Here's how the part is built. I have some questions about the finished solid (model axes, mm). A direction names the side the tool comes from. Give positions to 0.01 mm unless a question says otherwise; leave off trailing zeros. Write each loop counter-clockwise with the first axis right and the second up, starting at its lowest first coordinate (ties: lowest second). Pieces come first, ordered by that corner, then holes. Notation, with made-up numbers: (-21.5, -1) - (35.5, -1) arc R36 cw to (35.5, 37) - close; hole circle Ø4 at (74.5, 52). An arc over 180 degrees is marked (long way). Use one line per item in the form item = value. Start each with the question number.
from build123d import *

# Parameters (mm, degrees)
F1_DEPTH = 177.8
F2_R     = 12.7
F3_R     = 3.17499


# Not quite as in the source:
# - a fillet or chamfer is up to 0.001 mm smaller than in the source, because OpenCascade refuses the exact size


with BuildPart() as f1:
    # F0 (on Right) → F1 (new body, symmetric)
    with BuildSketch(Plane.YZ):
        Polygon((70.9975426912, -81.0872844047), (70.9975426912, 71.3127155953), (-81.4024573088, 71.3127155953), (-81.4024573088, -38.3387617767), (-62.3524573088, -49.3372844047), (-62.3524573088, -74.7372844047), (-81.4024573088, -74.7372844047), (-81.4024573088, -81.0872844047), align=None)
    extrude(amount=F1_DEPTH, both=True)

    # F2
    f2_edges = [f1.edges().sort_by_distance(p)[0] for p in [
        (0, -81.402457, -38.338762),
        (0, -81.402457, 71.312716),
        (0, 70.997543, 71.312716),
        (0, 70.997543, -81.087284),
    ]]
    fillet(f2_edges, radius=F2_R)

    # F3 (radius 3.175 in the source; OpenCascade refuses exactly that, so slightly less here)
    f3_edges = [f1.edges().sort_by_distance(p)[0] for p in [
        (0, -81.402457, -74.737284),
        (0, -81.402457, -81.087284),
    ]]
    fillet(f3_edges, radius=F3_R)


solid = f1.part
1. Please list where these lines run through material, in increasing order: line 1 (Y direction, x = -132.5, z = -55.5); line 2 (Z direction, x = 30, y = -72); line 3 (Y direction, x = 95, z = -71).
2. We'd pull the mould along Z, two halves only. Please class faces 1 (the face through (2.49, 67.38, 67.49)), 2 (the face through (2, -70, -74.737)), 3 (the face through (2, -62.352, -62)), 4 (the face through (2, -11, -81.087)): pulls with the +Z half, pulls with the -Z half, needs draft (parallel to the pull), parting line crosses it, or undercut.
3. For P1, Ø20.5, axis at x = 13, z = -60, coming from the -Y side; P2, Ø1.5, axis at x = 57.5, z = -42, coming from the -Y side, each with a flat end and sliding along its axis, tell me the tip position at first contact or that it passes through.
4. I want a section at B-B, the plane z = -59. List the corners of the cut face in (x, y) for me, then the cut area to 3 significant figures.
5. For faces 5 (the face through (2.49, -68.79, -45.62)), 6 (the face through (2, -81.402, 14)), which set-ups out of +Z, -Z, +X, -X, +Y, -Y let a thin tool reach every point of the face, with its end or its side?
Result sheet:
q1.line_1 = -62.35 to 71
q1.line_2 = -81.09 to -74.74, -43.77 to 70.88
q1.line_3 = -62.35 to 70.73
q2.face_1 = pulls with the +Z half
q2.face_2 = undercut
q2.face_3 = undercut
q2.face_4 = pulls with the -Z half
q3.P1 = -62.35
q3.P2 = -76.21
q4.outline = (-177.8, -62.35) - (177.8, -62.35) - (177.8, 71) - (-177.8, 71) - close
q4.area = 47,400 mm2
q5.face_5 = +X, -X, -Y
q5.face_6 = +Z, -Z, +X, -X, -Y
